Here's how the part is built. I have some questions about the finished solid (model axes, mm). Face numbers are marked on the shaded views. A direction names the side the tool comes from. Round coordinates to 2 decimals unless told otherwise and drop trailing zeros. Loops run counter-clockwise (first coordinate to the right, second up) from the corner with the lowest first, then second, coordinate; pieces in that order, holes last. Notation, with made-up numbers: M -28,37 L 5,37 A17 cw 5,50 Z; hole C -26,41.5 d9. An arc over 180 degrees is marked long. Write each question's results on one line, items separated by ' | '. Start each with the question number.
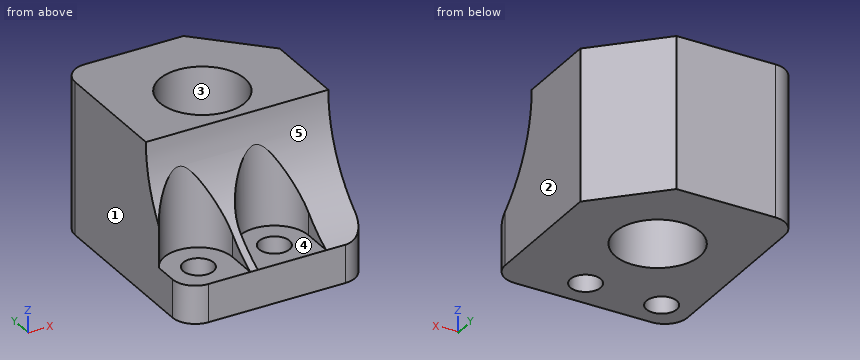
```python
from build123d import *

# Parameters (mm, degrees)
SKETCH1_R           = 2
SKETCH1_R_2         = 5.6
BOSS_EXTRUDE1_DEPTH = 20
CUT_EXTRUDE1_DEPTH  = 30
CUT_EXTRUDE2_DEPTH  = 15
FILLET1_R           = 3


with BuildPart() as part:
    # Sketch1 → Boss-Extrude1 (new body)
    with BuildSketch(Plane.XY):
        Polygon((24, 20), (16, 28), (0, 28), (0, 0), (24, 0), align=None)
        with Locations((4, 4)):
            Circle(SKETCH1_R, mode=Mode.SUBTRACT)
        with Locations((14, 4)):
            Circle(SKETCH1_R, mode=Mode.SUBTRACT)
        with Locations((11.5, 16)):
            Circle(SKETCH1_R_2, mode=Mode.SUBTRACT)
    extrude(amount=BOSS_EXTRUDE1_DEPTH)

    # Sketch2 → Cut-Extrude1 (cut)
    with BuildSketch(Plane.ZY):
        with BuildLine():
            Line((20, 9), (20, 0))
            Line((20, 0), (5, 0))
            ThreePointArc((5, 0), (11.253572158, 6.577379737), (20, 9))
        make_face()
    extrude(amount=-CUT_EXTRUDE1_DEPTH, mode=Mode.SUBTRACT)

    # Sketch3 → Cut-Extrude2 (cut)
    with BuildSketch(Plane.XY.offset(20)):
        with BuildLine():
            ThreePointArc((14, -0.5), (17.181980515, 0.818019485), (18.5, 4))
            Line((18.5, 4), (9.5, 4))
            ThreePointArc((9.5, 4), (10.818019485, 0.818019485), (14, -0.5))
        make_face()
        with BuildLine():
            Line((9.5, 4), (18.5, 4))
            ThreePointArc((18.5, 4), (14, 8.5), (9.5, 4))
        make_face()
        with BuildLine():
            ThreePointArc((14, -0.5), (10.818019485, 0.818019485), (9.5, 4))
            Line((9.5, 4), (9.5, -0.5))
            Line((9.5, -0.5), (14, -0.5))
        make_face()
        with BuildLine():
            Line((18.5, -0.5), (18.5, 4))
            ThreePointArc((18.5, 4), (17.181980515, 0.818019485), (14, -0.5))
            Line((14, -0.5), (18.5, -0.5))
        make_face()
        with BuildLine():
            ThreePointArc((4, -0.5), (7.181980515, 0.818019485), (8.5, 4))
            Line((8.5, 4), (0, 4))
            Line((0, 4), (0, 1.938447187))
            ThreePointArc((0, 1.938447187), (1.657670781, 0.157670781), (4, -0.5))
        make_face()
        with BuildLine():
            Line((0, 4), (8.5, 4))
            ThreePointArc((8.5, 4), (2.939339828, 8.373213921), (0, 1.938447187))
            Line((0, 1.938447187), (0, 4))
        make_face()
        with BuildLine():
            Line((8.5, -0.5), (8.5, 4))
            ThreePointArc((8.5, 4), (7.181980515, 0.818019485), (4, -0.5))
            Line((4, -0.5), (8.5, -0.5))
        make_face()
        with BuildLine():
            ThreePointArc((4, -0.5), (1.657670781, 0.157670781), (0, 1.938447187))
            Line((0, 1.938447187), (0, -0.5))
            Line((0, -0.5), (4, -0.5))
        make_face()
    extrude(amount=-CUT_EXTRUDE2_DEPTH, mode=Mode.SUBTRACT)

    # Fillet1
    fillet1_edges = [part.edges().sort_by_distance(p)[0] for p in [
        (0, 28, 10),
        (0, 0, 2.5),
        (24, 0, 2.5),
    ]]
    fillet(fillet1_edges, radius=FILLET1_R)


solid = part.part
```
1. If we mould it in two halves opening along X, with no side actions, what happens to the marked faces 1, 2 and 3? For each: released by +X, released by -X, zero draft, split by the parting line, or undercut.
2. I need wall thicknesses on line 1 along X through (y, z) = (4, 3.3); line 2 along Y through (x, z) = (4, 1.8); line 3 along Y through (x, z) = (11.5, 4.25). Which ranges of each line are inside material? Lowest first, please.
3. I want a section at A-A on x = 4. List the corners of the cut face in (y, z) for me, plus the area to 3 significant figures.
4. Which directions (+Z, -Z, +X, -X, +Y, -Y) give clear straight access to the entire face, cutting with the end or side of a thin tool? Please do the marked faces 4 and 5.
5. I want a section at B-B on z = 3.5. List the corners of the cut face in (x, y) for me.
6. I want a section at D-D on x = 14. List the corners of the cut face in (y, z) for me.
7. For pin 1 (5 mm diameter, centred on x = 4, y = 4, fed in from +Z); pin 2 (0.9 mm diameter, centred on y = 1, z = 6, fed in from -X); pin 3 (1.5 mm diameter, centred on y = 1.5, z = 5.5, fed in from +X), each with a flat end and sliding along its axis, tell me the tip position at first contact or that it passes through.
8. I want a section at C-C on y = 16. List the corners of the cut face in (x, z) for me.
Outcome:
1) face 1: released by -X | face 2: released by +X | face 3: undercut
2) line 1: 0 to 2, 6 to 12, 16 to 24 | line 2: 0 to 2, 6 to 28 | line 3: 0 to 10.4, 21.6 to 28
3) outline: M 0,0 L 2,0 L 2,5 L 0,5 Z; M 6,0 L 28,0 L 28,20 L 9,20 A17 cw 8.5,15.91 L 8.5,5 L 6,5 Z | area: 411 mm2
4) face 4: +Z, -Y | face 5: +Z, +X, -X, -Y
5) outline: M 0,3 A3 ccw 3,0 L 21,0 A3 ccw 24,3 L 24,20 L 16,28 L 3,28 A3 ccw 0,25 Z; hole C 4,4 d4; hole C 11.5,16 d11.2; hole C 14,4 d4
6) outline: M 0,0 L 2,0 L 2,5 L 0,5 Z; M 6,0 L 10.99,0 L 10.99,20 L 9,20 A17 cw 8.5,15.91 L 8.5,5 L 6,5 Z; M 21.01,0 L 28,0 L 28,20 L 21.01,20 Z
7) pin 1: z = 5 | pin 2: x = 8.5 | pin 3: x = 23.9
8) outline: M 0,0 L 5.9,0 L 5.9,20 L 0,20 Z; M 17.1,0 L 24,0 L 24,20 L 17.1,20 Z
